Verification items for the finished model (mm, model axes). A direction names the side the tool comes from. Give positions to 0.01 mm unless a question says otherwise; leave off trailing zeros. Loops run counter-clockwise (first coordinate to the right, second up) from the corner with the lowest first, then second, coordinate; pieces in that order, holes last. Notation, with made-up numbers: (7.25, -28.5) -> (29.25, -28.5) arc R15 ccw to (29.25, -1.5) -> close; hole circle Ø7 at (-37.75, 72.5). An arc over 180 degrees is marked (long way). Answer in a Markdown table with one row per item. Add a question column.
Q1. Section check B-B on x = 15. Enter the section's corners in (y, z), and give its area (3 significant figures).
Q2. Release check for a two-part mould opening along X. For faces 1 (the face through (13.79, 8.103, 3.042)), 2 (the face through (28, 10, 10)), 3 (the face through (0, 10, 4)) record: pulls with the +X half, pulls with the -X half, needs draft (parallel to the pull), parting line crosses it, or undercut.
Q3. Set-up check for faces 4 (the face through (28, 7.083, 8)), 5 (the face through (27, 13.083, 8)), 6 (the face through (3, 10, 10)), 7 (the face through (5.028, 10, 8)): record each of +Z, -Z, +X, -X, +Y, -Y from which the full face is reachable in a straight line by a thin tool's end or side.
Q4. Material ranges on probe 1 along X at (y, z) = (8.5, 8.5); probe 2 along Y at (x, z) = (15, 2.4); probe 3 along Z at (x, y) = (17.25, 7.25), recorded low to high.
Q5. Section check A-A on y = 10. Enter the section's corners in (x, z), and give its area (3 significant figures).
Q6. Gauge pin test, flat ends, axial feed: P1, Ø6, axis at x = 17.5, y = 2, coming from the +Z side; P2, Ø3, axis at x = 27.5, z = 8.5, coming from the -Y side. Record the tip position at first contact, or that the pin passes through.
Q7. Section check C-C on z = 8. Enter the section's corners in (x, y), and give its area (3 significant figures).
Q8. Section check D-D on z = 4.5. Enter the section's corners in (x, y), and give its area (3 significant figures).
Autodesk Fusion 360 part; units mm, degrees
sketch "Skizze1" plane through (0, 0, 0) normal (0, 0, 1) x (1, 0, 0)
  line L0 (0, 0) -> (30, 0)
  line L1 (30, 0) -> (30, 20)
  line L2 (30, 20) -> (0, 20)
  line L3 (0, 20) -> (0, 0)
  dimension "d1" = 30
  dimension "d2" = 20
extrude "Extrusion1" add sketch "Skizze1" along normal blind 6
sketch "Skizze2" plane through (0, 0, 6) normal (0, 0, 1) x (-1, 0, 0)
  line L0 (0, -20) -> (0, 0)
  line L1 (0, 0) -> (-30, 0)
  line L2 (-30, 0) -> (-30, -20)
  line L3 (-30, -20) -> (0, -20)
  line L4 (0, -13.0831) -> (-30, -13.0831)
  line L5 (-30, -13.0831) -> (-30, -7.0831)
  line L6 (-30, -7.0831) -> (0, -7.0831)
  line L7 (0, -7.0831) -> (0, -13.0831)
  dimension "d5" = 30
  dimension "d6" = 6
extrude "Extrusion2" add sketch "Skizze2" along normal blind 4 contours L0 L2 L4 L5 L6 L7
sketch "Skizze3" plane through (0, 0, 10) normal (0, 0, 1) x (-1, 0, 0)
  line L0 (0, -7.0831) -> (-30, -7.0831)
  line L1 (-30, -7.0831) -> (-30, -13.0831)
  line L2 (-30, -13.0831) -> (0, -13.0831)
  line L3 (0, -13.0831) -> (0, -7.0831)
  line L4 (-5.028, -13.0831) -> (-25.028, -13.0831)
  line L5 (-25.028, -13.0831) -> (-25.028, -7.0831)
  line L6 (-25.028, -7.0831) -> (-5.028, -7.0831)
  line L7 (-5.028, -7.0831) -> (-5.028, -13.0831)
  dimension "d9" = 20
  dimension "d10" = 6
extrude "Extrusion3" cut sketch "Skizze3" against normal blind 4 contours L0 L2 L4 L5 L6 L7
sketch "Skizze4" plane through (0, 0, 6) normal (0, 0, 1) x (-1, 0, 0)
  line L0 (0, -13.0831) -> (-5.028, -13.0831)
  line L1 (-5.028, -13.0831) -> (-5.028, -7.0831)
  line L2 (-5.028, -7.0831) -> (0, -7.0831)
  line L3 (0, -7.0831) -> (0, 0)
  line L4 (0, 0) -> (-30, 0)
  line L5 (-30, 0) -> (-30, -7.0831)
  line L6 (-30, -7.0831) -> (-25.028, -7.0831)
  line L7 (-25.028, -7.0831) -> (-25.028, -13.0831)
  line L8 (-25.028, -13.0831) -> (-30, -13.0831)
  line L9 (-30, -13.0831) -> (-30, -20)
  line L10 (-30, -20) -> (0, -20)
  line L11 (0, -20) -> (0, -13.0831)
  circle A0 centre (-15, -10) radius 2.25
  dimension "d13" = 4.5
extrude "Extrusion4" cut sketch "Skizze4" against normal blind 6 contours A0
Taken from the geometry:
| question | item | result |
|---|---|---|
| 1 | outline | (0, 0) -> (7.75, 0) -> (7.75, 6) -> (0, 6) -> close; (12.25, 0) -> (20, 0) -> (20, 6) -> (12.25, 6) -> close |
| 1 | area | 93.0 mm² |
| 2 | face 1 | undercut |
| 2 | face 2 | needs draft |
| 2 | face 3 | pulls with the -X half |
| 3 | face 4 | +Z, +X, -X, -Y |
| 3 | face 5 | +Z, +X, -X, +Y |
| 3 | face 6 | +Z, +X, -X, +Y, -Y |
| 3 | face 7 | +Z, +Y, -Y |
| 4 | probe 1 | x = 0 to 5.03, 25.03 to 30 |
| 4 | probe 2 | y = 0 to 7.75, 12.25 to 20 |
| 4 | probe 3 | z = 0 to 6 |
| 5 | outline | (0, 0) -> (12.75, 0) -> (12.75, 6) -> (5.03, 6) -> (5.03, 10) -> (0, 10) -> close; (17.25, 0) -> (30, 0) -> (30, 10) -> (25.03, 10) -> (25.03, 6) -> (17.25, 6) -> close |
| 5 | area | 193 mm² |
| 6 | P1 | stops at z = 6 |
| 6 | P2 | stops at y = 7.08 |
| 7 | outline | (0, 7.08) -> (5.03, 7.08) -> (5.03, 13.08) -> (0, 13.08) -> close; (25.03, 7.08) -> (30, 7.08) -> (30, 13.08) -> (25.03, 13.08) -> close |
| 7 | area | 60.0 mm² |
| 8 | outline | (0, 0) -> (30, 0) -> (30, 20) -> (0, 20) -> close; hole circle Ø4.5 at (15, 10) |
| 8 | area | 584 mm² |
